Answer from the drawing. Dimensions are ordinates in mm from the lowest x, y and z of the part. A direction names the side the tool comes from. Round coordinates to 2 decimals unless told otherwise and drop trailing zeros. Write each loop counter-clockwise with the first axis right and the second up, starting at its lowest first coordinate (ties: lowest second). Pieces come first, ordered by that corner, then holes. Notation, with made-up numbers: (89, -22) - (102, -22) arc R16 ccw to (102, -16) - close; hole circle Ø1 at (31, -4). An arc over 180 degrees is marked (long way). Answer as CSV lines item,"result". Start each with the question number.
1) Consider line 1 along Z through (x, y) = (11.5, 19.5); line 2 along X through (y, z) = (11.75, 9.25); line 3 along Y through (x, z) = (11.5, 17.5). Determine where each line is inside the solid, lowest interval first.
2) Find section B-B on x = 11.5. Determine the outline of the cut face in (y, z), then the cut area to 3 significant figures.
3) Which of the six approach directions +Z, -Z, +X, -X, +Y, -Y give full straight-line access (tool end or side, diameter ignored) to the marked faces 1 and 2?
4) Find section C-C on z = 21.4. Determine the outline of the cut face in (x, y).
5) Find section D-D on y = 14.5. Determine the outline of the cut face in (x, z), then the cut area to 3 significant figures.
6) Each of these flat-tipped pins is pushed along its axis until it touches: pin 1 (6 mm diameter, centred on x = 18.5, z = 15, fed in from -Y); pin 2 (4 mm diameter, centred on x = 9, z = 12, fed in from +Y); pin 3 (4.5 mm diameter, centred on x = 11.5, y = 11.5, fed in from -Z); pin 4 (10 mm diameter, centred on x = 16.5, z = 9, fed in from -Y). Where does it stop, or does it pass through?
7) Find section A-A on y = 11.5. Determine the outline of the cut face in (x, z).
8) For a pull along X with two mould halves and no side action, classify the marked faces 3, 4, 5 and 6 as +X half, -X half, draft (parallel to the pull), parting line (faces both ways), or undercut.
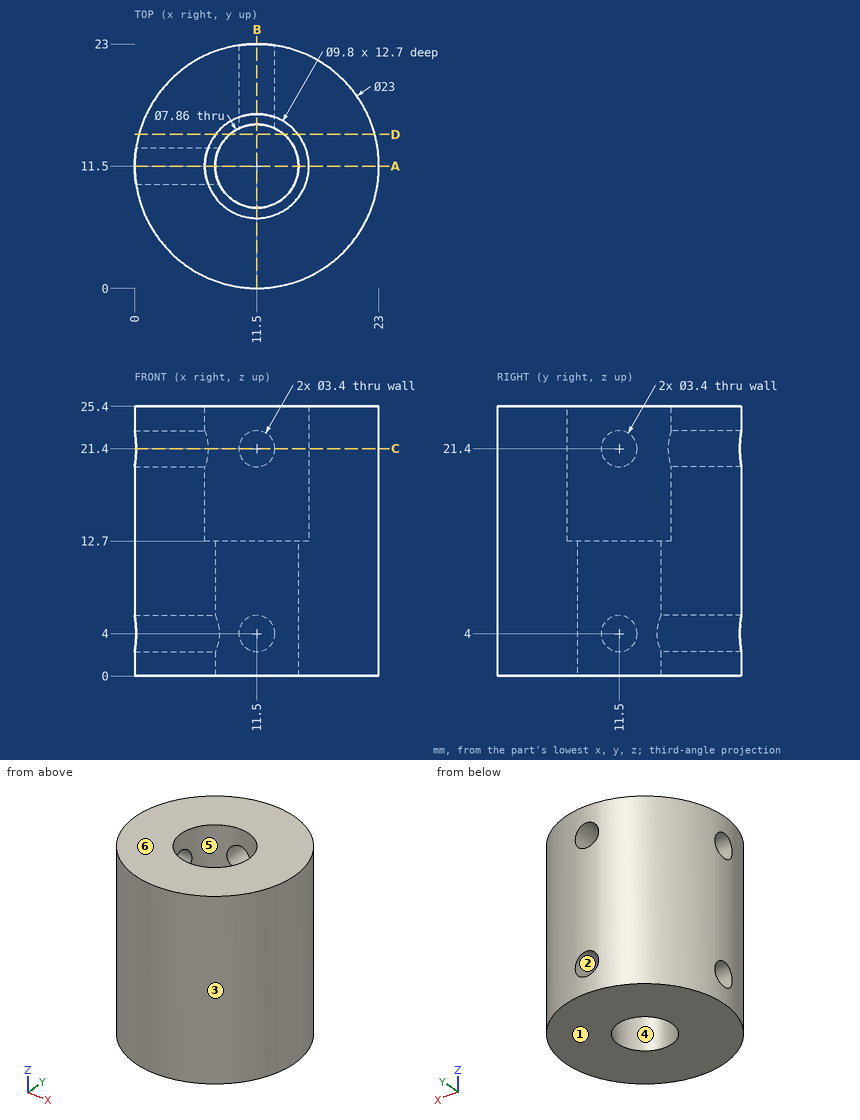
Check values:
1,line 1,"z = 0 to 2.3, 5.7 to 19.7, 23.1 to 25.4"
1,line 2,"x = 0 to 7.58, 15.42 to 23"
1,line 3,"y = 0 to 6.6, 16.4 to 23"
2,outline,"(0, 0) - (7.57, 0) - (7.57, 12.7) - (6.6, 12.7) - (6.6, 25.4) - (0, 25.4) - close; (15.43, 0) - (23, 0) - (23, 2.3) - (15.43, 2.3) - close; (15.43, 5.7) - (23, 5.7) - (23, 19.7) - (16.4, 19.7) - (16.4, 12.7) - (15.43, 12.7) - close; (16.4, 23.1) - (23, 23.1) - (23, 25.4) - (16.4, 25.4) - close"
2,area,"312 mm^2"
3,face 1,"-Z, +X, -X, +Y, -Y"
3,face 2,"+Y"
4,outline,"(0.13, 9.8) arc R11.5 ccw (long way) to (13.2, 22.87) - (13.2, 16.1) arc R4.9 cw (long way) to (6.9, 9.8) - close; (0.13, 13.2) - (6.9, 13.2) arc R4.9 cw to (9.8, 16.1) - (9.8, 22.87) arc R11.5 ccw to start"
5,outline,"(0.4, 0) - (8.96, 0) - (8.96, 12.7) - (7.63, 12.7) - (7.63, 25.4) - (0.4, 25.4) - close; (14.04, 0) - (22.6, 0) - (22.6, 25.4) - (15.37, 25.4) - (15.37, 12.7) - (14.04, 12.7) - close"
5,area,"401 mm^2"
6,pin 1,"stops at y = 0.72"
6,pin 2,"stops at y = 22.99"
6,pin 3,"passes through"
6,pin 4,"stops at y = 0"
7,outline,"(0, 0) - (7.57, 0) - (7.57, 2.3) - (0, 2.3) - close; (0, 5.7) - (7.57, 5.7) - (7.57, 12.7) - (6.6, 12.7) - (6.6, 19.7) - (0, 19.7) - close; (0, 23.1) - (6.6, 23.1) - (6.6, 25.4) - (0, 25.4) - close; (15.43, 0) - (23, 0) - (23, 25.4) - (16.4, 25.4) - (16.4, 12.7) - (15.43, 12.7) - close"
8,face 3,"parting line"
8,face 4,"undercut"
8,face 5,"undercut"
8,face 6,"draft"
